The model under review builds one solid part; all positions refer to its coordinate system, in mm. A direction names the side the tool comes from. Give positions to 0.01 mm unless a question says otherwise; leave off trailing zeros. Loops run counter-clockwise (first coordinate to the right, second up) from the corner with the lowest first, then second, coordinate; pieces in that order, holes last. Notation, with made-up numbers: M -25.75,-24 L 32.25,-24 A13 ccw 32.25,-20 Z; hole C 33.5,-1.5 d6. An arc over 180 degrees is marked long. Write item = value, one per line. Start each with the question number.
1. We need section A-A on z = 1.15. Count the separate pieces of the cut face and the enclosed holes in it, then the cut area to 3 significant figures.
2. We need section B-B on y = 0. Give the boundary of the cut face in (x, z) (3 decimals).
3. We need section C-C on y = 10.5. Give the boundary of the cut face in (x, z).
4. For faces 1 (the face through (48.61, 5.2, 1.48)), 2 (the face through (25, 3, 3)), list the 3-axis set-ups (+Z, -Z, +X, -X, +Y, -Y) from which the entire face can be reached by the end or side of a thin tool; tool diameter is ignored.
5. For pin 1 (1.5 mm diameter, centred on x = 11, z = 1, fed in from +Y); pin 2 (1 mm diameter, centred on x = 34.5, z = 2.5, fed in from -Y); pin 3 (2.5 mm diameter, centred on x = 0, y = 0, fed in from +Z), all flat-tipped, find the tip position at first contact; note any pin that passes through.
6. We need section D-D on x = 24.5. Give the boundary of the cut face in (y, z), then the cut area to 3 significant figures.
7. Wall thickness on line 1 along Y through (x, z) = (0, 2.15) (3 decimals); line 2 along Y through (x, z) = (22, 0.8) (3 decimals); line 3 along X through (y, z) = (-0.5, 1.7): over which ranges is each line inside the solid? List them lowest first. Write a range as from..to.
8. Draft analysis for pull direction X (two halves, no side actions). For faces 3 (the face through (-5, 0, 1)), 4 (the face through (52.312, 6.722, 1.479)), 5 (the face through (55.3, 8.4, 1.5)), 6 (the face through (10, 5, 1)), state which applies: pulls with the +X half, pulls with the -X half, needs draft (parallel to the pull), parting line crosses it, or undercut.
from build123d import *

# Parameters (mm, degrees)
SKETCH1_R           = 1.525
BOSS_EXTRUDE1_DEPTH = 3
FILLET1_R           = 1


with BuildPart() as part:
    # Sketch1 → Boss-Extrude1 (new body)
    # profile 1 of 2: a face of its own
    with BuildSketch(Plane.XY):
        with BuildLine():
            Line((20.05, 5), (0, 5))
            ThreePointArc((0, 5), (-5, 0), (0, -5))
            Line((0, -5), (22, -5))
            Line((22, -5), (26.644435765, 1.851814361))
            ThreePointArc((26.644435765, 1.851814361), (24.805434743, 4.138784351), (22, 5))
            Line((22, 5), (20.05, 5))
        make_face()
        Circle(SKETCH1_R, mode=Mode.SUBTRACT)
        with Locations((22, 0)):
            Circle(SKETCH1_R, mode=Mode.SUBTRACT)
    # profile 2 of 2: a face of its own
    with BuildSketch(Plane.XY):
        with BuildLine():
            Line((46.409029503, 15.837507263), (20.05, 5))
            Line((20.05, 5), (22, 5))
            ThreePointArc((22, 5), (24.805434743, 4.138784351), (26.644435765, 1.851814361))
            Line((26.644435765, 1.851814361), (39.871788822, 7.125781662))
            Line((39.871788822, 7.125781662), (46.188488025, 4.540007042))
            Line((46.188488025, 4.540007042), (47.352932204, 4.337597171))
            Line((47.352932204, 4.337597171), (48.038244482, 5.300533868))
            Line((48.038244482, 5.300533868), (49.20268866, 5.098123997))
            Line((49.20268866, 5.098123997), (49.888000938, 6.061060693))
            Line((49.888000938, 6.061060693), (51.052445116, 5.858650822))
            Line((51.052445116, 5.858650822), (51.737757394, 6.821587519))
            Line((51.737757394, 6.821587519), (52.902201573, 6.619177648))
            Line((52.902201573, 6.619177648), (53.587513851, 7.582114344))
            Line((53.587513851, 7.582114344), (54.751958029, 7.379704473))
            Line((54.751958029, 7.379704473), (55.437270307, 8.34264117))
            Line((55.437270307, 8.34264117), (53.72608495, 12.504593197))
            Line((53.72608495, 12.504593197), (46.409029503, 15.837507263))
        make_face()
    extrude(amount=BOSS_EXTRUDE1_DEPTH)

    # Fillet1
    fillet1_edges = [part.edges().sort_by_distance(p)[0] for p in [
        (22, -5, 1.5),
        (20.05, 5, 1.5),
        (46.409029503, 15.837507263, 1.5),
        (53.72608495, 12.504593197, 1.5),
        (55.437270307, 8.34264117, 1.5),
        (46.188488025, 4.540007042, 1.5),
        (39.871788822, 7.125781662, 1.5),
        (26.644435765, 1.851814361, 1.5),
    ]]
    fillet(fillet1_edges, radius=FILLET1_R)


solid = part.part
Final values:
q1.separate_pieces = 1
q1.enclosed_holes = 2
q1.area = 486 mm²
q2.outline = M -5,0 L -1.525,0 L -1.525,3 L -5,3 Z; M 1.525,0 L 20.475,0 L 20.475,3 L 1.525,3 Z; M 23.525,0 L 25.389,0 L 25.389,3 L 23.525,3 Z
q3.outline = M 33.43,0 L 54.55,0 L 54.55,3 L 33.43,3 Z
q4.face_1 = +Z, -Z, -Y
q4.face_2 = +Z, +X, -X, +Y, -Y
q5.pin_1 = 5
q5.pin_2 = 4.78
q5.pin_3 = through
q6.outline = M -1.31,0 L 6.83,0 L 6.83,3 L -1.31,3 Z
q6.area = 24.4 mm²
q7.line_1 = -5..-1.525, 1.525..5
q7.line_2 = -4.848..-1.525, 1.525..5.802
q7.line_3 = -4.97..-1.44, 1.44..20.56, 23.44..25.05
q8.face_3 = pulls with the -X half
q8.face_4 = undercut
q8.face_5 = pulls with the +X half
q8.face_6 = needs draft
